Autodesk Inventor part; units mm, degrees
ref_plane "YZ Plane" through (0, 0, 0) normal (1, 0, 0) x (0, 1, 0)
ref_plane "XZ Plane" through (0, 0, 0) normal (0, 1, 0) x (-1, 0, 0)
ref_plane "XY Plane" through (0, 0, 0) normal (0, 0, 1) x (1, 0, 0)
sketch "Sketch1" plane through (0, 0, 0) normal (1, 0, 0) x (0, 1, 0)
  line L0 (0, -315) -> (0, 0)
  line L1 (-60, -315) -> (0, -315)
  line L2 (-60, -315) -> (-60, -242.7852)
  line L3 (-60, -242.7852) -> (-230, 0)
  line L4 (-230, 0) -> (0, 0)
  line L5 (-204.5995, -31.0454) -> (-193.128, -47.4284)
  line L6 (-193.128, -47.4284) -> (-195.5854, -49.1491)
  line L7 (-195.5854, -49.1491) -> (-207.0569, -32.7661)
  line L8 (-207.0569, -32.7661) -> (-204.5995, -31.0454)
  line L9 (-230, -17.4345) -> (-60, -260.2196)
  line L10 (-230, 0) -> (-230, -17.4345)
  point P0 (-45, -305)
  point P1 (-201.3212, -40.9576)
  point P2 (-198.8637, -39.2369)
  dimension "d0" = 60
  dimension "d7" = 15
  dimension "d47" = 315
  dimension "d48" = 230
  dimension "d49" = 55
  dimension "d51" = 3
  dimension "d52" = 20
  dimension "d54" = 40
  dimension "d59" = 10
  dimension "d60" = 0
  dimension "d63" = 10
extrude "Extrusion1" add sketch "Sketch1" along normal mid plane 3
sketch "Sketch2" plane through (1.5, 0, 0) normal (1, 0, 0) x (0, 0, -1)
  line L0 (29.3246, -202.142) -> (45.7077, -190.6705)
  line L1 (45.7077, -190.6705) -> (43.9869, -188.213)
  line L2 (43.9869, -188.213) -> (27.6039, -199.6846)
  line L3 (27.6039, -199.6846) -> (29.3246, -202.142)
  line L4 (0, 0) -> (0, -230) construction
  line L5 (17.4345, -230) -> (260.2196, -60)
  line L6 (29.3246, -202.142) -> (0, -221.4287) construction
  dimension "d24" = 3
  dimension "d25" = 20
  dimension "d55" = 40
  dimension "d61" = 16
  dimension "d67" = 35.0986
extrude "Extrusion2" cut sketch "Sketch2" against normal blind 3
pattern_linear "Rectangular Pattern1" count 5 spacing 60 along (0, 0.5736, -0.8192) of "Extrusion2"
sketch "Sketch3" plane through (1.5, 0, 0) normal (1, 0, 0) x (0, 0, -1)
  line L0 (315, -60) -> (315, 0)
  line L1 (315, 0) -> (0, 0)
  line L2 (260.2196, -60) -> (315, -60)
  point P0 (300, -45)
  dimension "d64" = 15
  dimension "d65" = 15
hole "Hole3" at (1.5, -45, -300) direction (-1, 0, 0) diameter 4.134 end through all
fillet "Fillet1" radius 40 1 edges at (0, 0, 0)
properties part number "2309HCMUTE-CDT23_VACH-NGAN" material "PMMA Plastic"
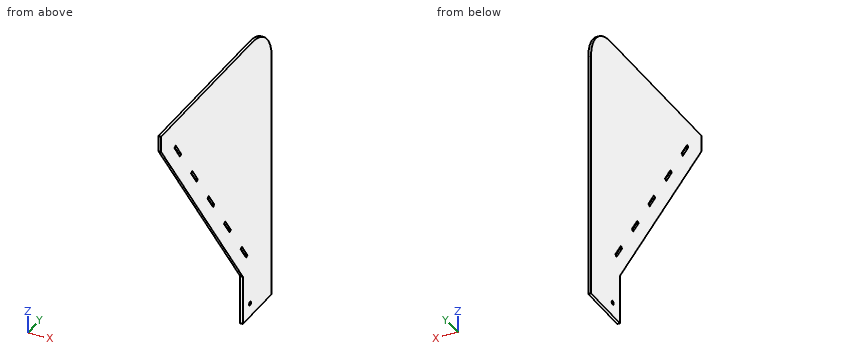
Could you check a few things on this model? Use its own coordinates, in mm. Coordinates: 2 decimals unless noted, no trailing zeros. Write each loop counter-clockwise with the first axis right and the second up, starting at its lowest first coordinate (ties: lowest second). Pieces come first, ordered by that corner, then holes. Notation, with made-up numbers: (-3, -25.5) - (32, -25.5) arc R32 cw to (32, 6.5) - close; hole circle Ø9 at (84.5, -0.5). An arc over 180 degrees is marked (long way). Use a Markdown table: item, result.
Q1. Imagine slicing it at A-A (x = 1.05). List the corners of the cut face in (y, z) for me, and give its area (3 significant figures).
Geometry check:
| item | result |
|---|---|
| outline | (-230, -17.43) - (-60, -260.22) - (-60, -315) - (0, -315) - (0, -40) arc R40 ccw to (-40, 0) - (-230, 0) - close; hole (-202.14, -29.32) - (-190.67, -45.71) - (-188.21, -43.99) - (-199.68, -27.6) - close; hole (-167.73, -78.47) - (-156.26, -94.86) - (-153.8, -93.14) - (-165.27, -76.75) - close; hole (-133.31, -127.62) - (-121.84, -144.01) - (-119.38, -142.29) - (-130.86, -125.9) - close; hole (-98.9, -176.77) - (-87.43, -193.16) - (-84.97, -191.43) - (-96.44, -175.05) - close; hole (-64.48, -225.92) - (-53.01, -242.3) - (-50.55, -240.58) - (-62.03, -224.2) - close; hole circle Ø4.13 at (-45, -300) |
| area | 41,800 mm2 |
Q2. Please list where these lines run through material, in increasing order: L1, parallel to Y at x = -0.4, z = -300; L2, parallel to Z at x = -0.15, y = -45; L3, parallel to Z at x = 0.7, y = -193.
Geometry check:
| item | result |
|---|---|
| L1 | y = -60 to -47.07, -42.93 to 0 |
| L2 | z = -315 to -302.07, -297.93 to 0 |
| L3 | z = -70.28 to -42.38, -37.15 to 0 |
Q3. Imagine slicing it at C-C (z = -133). List the corners of the cut face in (x, y) for me.
Geometry check:
| item | result |
|---|---|
| outline | (-1.5, -149.08) - (1.5, -149.08) - (1.5, -129.55) - (-1.5, -129.55) - close; (-1.5, -125.89) - (1.5, -125.89) - (1.5, 0) - (-1.5, 0) - close |
Q4. I'm going to push flat-ended pins straight in: pin 1 Ø1.5 at (x, z) = (0.5, -170) entering from -Y; pin 2 Ø1.5 at (x, y) = (-0.5, -120) entering from -Z. Where does each tip first touch, or does it pass through?
Geometry check:
| item | result |
|---|---|
| pin 1 | stops at y = -123.7 |
| pin 2 | stops at z = -175.6 |
Q5. Imagine slicing it at D-D (y = -184). List the corners of the cut face in (x, z) for me, and give its area (3 significant figures).
Geometry check:
| item | result |
|---|---|
| outline | (-1.5, -83.13) - (1.5, -83.13) - (1.5, 0) - (-1.5, 0) - close |
| area | 249 mm2 |
Q6. Imagine slicing it at B-B (z = -83). List the corners of the cut face in (x, y) for me.
Geometry check:
| item | result |
|---|---|
| outline | (-1.5, -184.09) - (1.5, -184.09) - (1.5, -164.56) - (-1.5, -164.56) - close; (-1.5, -160.9) - (1.5, -160.9) - (1.5, 0) - (-1.5, 0) - close |
